Work out the finished part from the listing and answer in its coordinate system (mm). A direction names the side the tool comes from. Give positions to 0.01 mm unless a question says otherwise; leave off trailing zeros. Loops run counter-clockwise (first coordinate to the right, second up) from the corner with the lowest first, then second, coordinate; pieces in that order, holes last.
```python
from build123d import *

# Parameters (mm, degrees)
SKETCH1_R           = 6.5
BOSS_EXTRUDE1_DEPTH = 8
CUT_EXTRUDE1_DEPTH  = 4
SKETCH3_R           = 4
BOSS_EXTRUDE2_DEPTH = 100


with BuildPart() as part:
    # Sketch1 → Boss-Extrude1 (new body)
    with BuildSketch(Plane.YZ):
        with Locations(Location((0, 0, 0), (0, 0, 270))):
            Circle(SKETCH1_R)
    extrude(amount=BOSS_EXTRUDE1_DEPTH)

    # Sketch2 → Cut-Extrude1 (cut)
    with BuildSketch(Plane(origin=(0, 0, 0), x_dir=(0, -1, 0), z_dir=(-1, 0, 0))):
        Polygon((3.464101615, 0), (1.732050808, 3), (-1.732050808, 3), (-3.464101615, 0), (-1.732050808, -3), (1.732050808, -3), align=None)
    extrude(amount=-CUT_EXTRUDE1_DEPTH, mode=Mode.SUBTRACT)

    # Sketch3 → Boss-Extrude2 (add)
    with BuildSketch(Plane.YZ.offset(8)):
        with Locations(Location((0, 0, 0), (0, 0, 270))):
            Circle(SKETCH3_R)
    extrude(amount=BOSS_EXTRUDE2_DEPTH)


solid = part.part
```
Q1. Section B-B on x = 56 is taken. Give the vertices of the cut face in (y, z), plus the area to 3 significant figures.
Q2. Determine the mould class of faces 4 (the face through (2, 2.6, 1.5)), 5 (the face through (3.944, -3.955, 5.158)), 6 (the face through (8, 3, -3)), 7 (the face through (2, 0, 3)) for opening direction Y: +Y half, -Y half, draft (parallel to the pull), parting line (faces both ways), or undercut.
Q3. Section A-A on y = 0 is taken. Give the vertices of the cut face in (x, z), plus the area to 3 significant figures.
Q4. Section D-D on z = 5.5 is taken. Give the vertices of the cut face in (x, y), plus the area to 3 significant figures.
Q5. Which of the six approach directions +Z, -Z, +X, -X, +Y, -Y give full straight-line access (tool end or side, diameter ignored) to faces 1 (the face through (57.3, -3.905, 0.867)), 2 (the face through (108, 0, 0)), 3 (the face through (2, 2.6, -1.5))?
Q6. Section C-C on z = 1.5 is taken. Give the vertices of the cut face in (x, y), plus the area to 3 significant figures.
Q7. Given pin 1 (1 mm diameter, centred on x = 19.5, z = 4, fed in from +Y); pin 2 (3 mm diameter, centred on x = 85, y = -3, fed in from -Z); pin 3 (3 mm diameter, centred on x = 62, y = -1.5, fed in from -Z), each flat-ended and moving along its own axis, determine where each tip first touches the part or whether it passes through.
Q8. Consider line 1 along X through (y, z) = (5, 2); line 2 along Z through (x, y) = (90.5, 2); line 3 along Z through (x, y) = (41, -3). Determine where each line is inside the solid, lowest interval first.
Check result:
1. outline: circle Ø8 at (0, 0)
1. area: 50.3 mm2
2. face 4: undercut
2. face 5: parting line
2. face 6: draft
2. face 7: undercut
3. outline: (0, -6.5) - (8, -6.5) - (8, -4) - (108, -4) - (108, 4) - (8, 4) - (8, 6.5) - (0, 6.5) - (0, 3) - (4, 3) - (4, -3) - (0, -3) - close
3. area: 880 mm2
4. outline: (0, -3.46) - (8, -3.46) - (8, 3.46) - (0, 3.46) - close
4. area: 55.4 mm2
5. face 1: +X
5. face 2: +Z, -Z, +X, +Y, -Y
5. face 3: -X
6. outline: (0, -6.32) - (8, -6.32) - (8, -3.71) - (108, -3.71) - (108, 3.71) - (8, 3.71) - (8, 6.32) - (0, 6.32) - (0, 2.6) - (4, 2.6) - (4, -2.6) - (0, -2.6) - close
6. area: 822 mm2
7. pin 1: stops at y = 1.94
7. pin 2: stops at z = -3.71
7. pin 3: stops at z = -4
8. line 1: x = 0 to 8
8. line 2: z = -3.46 to 3.46
8. line 3: z = -2.65 to 2.65
